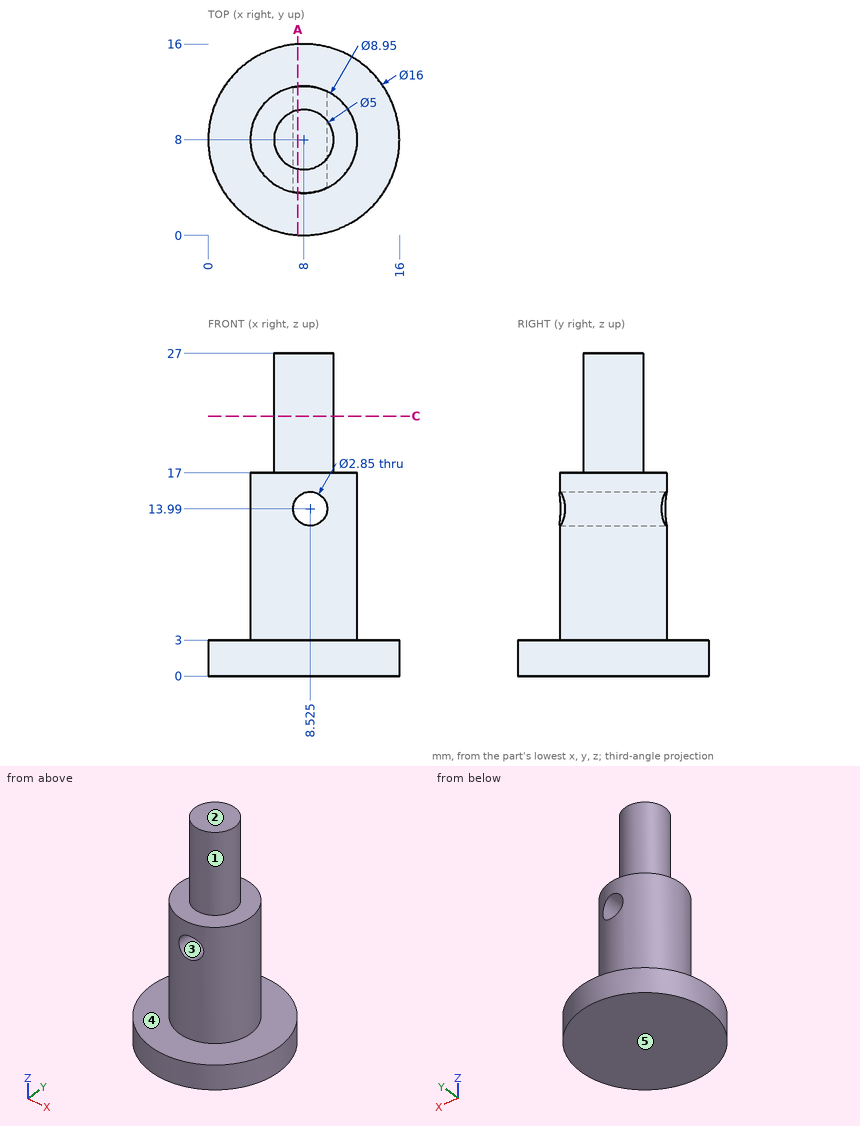
Geometry: see drawing. Coordinates: mm, zero at the bounding-box minimum. A direction names the side the tool comes from. Give positions to 0.01 mm unless a question says otherwise; leave off trailing zeros. Order: outer loops, then holes, each group sorted by start corner. A loop starts at its lowest first (then second) coordinate and runs counter-clockwise, first axis right, second up. Notation, with made-up numbers: (28.25, -16) - (46.25, -16) arc R21 ccw to (46.25, 5) - close; hole circle Ø10 at (11, -26.5). An arc over 180 degrees is marked (long way). Use CSV: the item, a comma, the result in double quotes.
1. Material intervals for line 1 along Z through (x, y) = (1.5, 3.5); line 2 along Z through (x, y) = (8, 8.5) (1 decimal); line 3 along X through (y, z) = (8.5, 11.75), sorted ascending. Write a range as from..to.
Answers below:
line 1,"0..3"
line 2,"0..12.7, 15.3..27"
line 3,"3.55..12.45"
2. Section query A-A (x = 7.5). Output: boundary loops of the cut face in (y, z), plus the area to 3 significant figures.
Answers below:
outline,"(0.02, 0) - (15.98, 0) - (15.98, 3) - (12.45, 3) - (12.45, 13) - (3.55, 13) - (3.55, 3) - (0.02, 3) - close; (3.55, 14.98) - (12.45, 14.98) - (12.45, 17) - (10.45, 17) - (10.45, 27) - (5.55, 27) - (5.55, 17) - (3.55, 17) - close"
area,"204 mm2"
3. Access query for the marked faces 4 and 5. Directions: +Z, -Z, +X, -X, +Y, -Y. A direction counts if a zero-diameter tool reaches every point of the face in a straight line with its end or side. Return the directions, or none.
Answers below:
face 4,"+Z"
face 5,"-Z, +X, -X, +Y, -Y"
4. Mould query, pull axis X, two halves, no side actions, for the marked faces 1, 2 and 3. Classes: +X half, -X half, draft (parallel to the pull), parting line (faces both ways), or undercut.
Answers below:
face 1,"parting line"
face 2,"draft"
face 3,"undercut"
5. Section query C-C (z = 21.75). Output: boundary loops of the cut face in (x, y), plus the area to 3 significant figures.
Answers below:
outline,"circle Ø5 at (8, 8)"
area,"19.6 mm2"
6. Contact query for flat-ended pins moving along their axis: pin 1 (3 mm diameter, centred on x = 6, y = 13.5, fed in from +Z); pin 2 (4 mm diameter, centred on y = 8.5, z = 23.5, fed in from +X); pin 3 (5 mm diameter, centred on y = 9, z = 13, fed in from +X) (3 decimals). Output: stop coordinate, or through.
Answers below:
pin 1,"z = 17"
pin 2,"x = 10.5"
pin 3,"x = 12.475"
